```python
from build123d import *

# Parameters (mm, degrees)
SKETCH1_R           = 9
BOSS_EXTRUDE1_DEPTH = 70
SKETCH2_R           = 2.5
CUT_EXTRUDE1_DEPTH  = 15
CUT_EXTRUDE2_START  = -50
SKETCH3_R           = 9
SKETCH3_R_2         = 7.5
CUT_EXTRUDE2_DEPTH  = 50
FILLET1_R           = 10


with BuildPart() as part:
    # Sketch1 → Boss-Extrude1 (new body)
    with BuildSketch(Plane.XY):
        Circle(SKETCH1_R)
    extrude(amount=BOSS_EXTRUDE1_DEPTH)

    # Sketch2 → Cut-Extrude1 (cut)
    with BuildSketch(Plane(origin=(0, 0, 0), x_dir=(-1, 0, 0), z_dir=(0, 0, -1))):
        Circle(SKETCH2_R)
    extrude(amount=-CUT_EXTRUDE1_DEPTH, mode=Mode.SUBTRACT)

    # Sketch3 → Cut-Extrude2 (cut)
    with BuildSketch(Plane.XY.offset(70).offset(CUT_EXTRUDE2_START)):
        Circle(SKETCH3_R)
        Circle(SKETCH3_R_2, mode=Mode.SUBTRACT)
    extrude(amount=CUT_EXTRUDE2_DEPTH, mode=Mode.SUBTRACT)

    # Fillet1
    # the kernel refuses this fillet: 10 mm, written as the material it adds along each edge
    with BuildSketch(Plane(origin=(0, 0, 20), x_dir=(1, 0, 0), z_dir=(0, -1, 0))) as fillet1_piece_1:
        with BuildLine():
            CenterArc((17.5, 5.267826876), FILLET1_R, 180, 31.788330617)
            Line((7.5, 5.267826876), (7.3, 5.267826876))
            Line((7.3, 5.267826876), (7.3, 0))
            Line((7.3, 0), (7.5, -0.2))
            ThreePointArc((7.5, -0.2), (8.25, -0.2), (8.83, -0.105356538))
            Line((8.83, -0.105356538), (9, 0))
        make_face()
    revolve(axis=Axis((0, 0, 20), (0, 0, 1)))


solid = part.part
```
Model file for the job. Use its own axes, mm. A direction names the side the tool comes from. Coordinates: 2 decimals unless noted, no trailing zeros. Write each loop counter-clockwise with the first axis right and the second up, starting at its lowest first coordinate (ties: lowest second). Pieces come first, ordered by that corner, then holes. Notation, with made-up numbers: (15, 42.5) - (20, 42.5) arc R23 cw to (20, 79.5) - close; hole circle Ø10 at (4, 41.25). An arc over 180 degrees is marked (long way). One line per question, with ' | ' between items. Start each with the question number.
Q1. Cut at A-A, the plane y = 0. List the corners of the cut face in (x, z).
Q2. Drill centre lines: line 1 (Y direction, x = 0, z = 8.5); line 2 (Z direction, x = 1.25, y = -2); line 3 (X direction, y = -2, z = 7.5). Where is each one in solid material? Low to high. Write a range as [from, to].
Q3. Pull direction X, two halves, no side cores. Call faces 3 (the face through (-7.493, 0.33, 47.321)), 4 (the face through (2, -2, 0)), 5 (the face through (0, 0, 15)): pulls with the +X half, pulls with the -X half, needs draft (parallel to the pull), parting line crosses it, or undercut.
Q4. Cut at C-C, the plane z = 66.5. List the corners of the cut face in (x, y).
Q5. Cut at D-D, the plane z = 10.5. List the corners of the cut face in (x, y), then the cut area to 3 significant figures.
Q6. Pin check, flat tips, straight feed: pin 1 (2 mm diameter, centred on y = 6.5, z = 46.5, fed in from +X); pin 2 (1 mm diameter, centred on x = -3, z = 61, fed in from +Y); pin 3 (5 mm diameter, centred on y = 0.5, z = 37.5, fed in from -X); pin 4 (6 mm diameter, centred on x = 0, y = 0, fed in from -Z). Stop position of each tip, or through.
Q7. 3-axis set-ups, long thin cutter, end or side, ignore diameter. For faces 1 (the face through (0.54, -2.44, 7.4)), 2 (the face through (0, 0, 70)): which of +Z, -Z, +X, -X, +Y, -Y reach the whole face in a straight line?
Answer below:
1) outline: (-9, 0) - (-2.5, 0) - (-2.5, 15) - (2.5, 15) - (2.5, 0) - (9, 0) - (9, 20) arc R10 cw to (7.5, 25.27) - (7.5, 70) - (-7.5, 70) - (-7.5, 25.27) arc R10 cw to (-9, 20) - close
2) line 1: [-9, -2.5], [2.5, 9] | line 2: [15, 70] | line 3: [-8.77, -1.5], [1.5, 8.77]
3) face 3: parting line crosses it | face 4: needs draft | face 5: undercut
4) outline: circle Ø15 at (0, 0)
5) outline: circle Ø18 at (0, 0); hole circle Ø5 at (0, 0) | area: 235 mm^2
6) pin 1: x = 5.1 | pin 2: y = 7.07 | pin 3: x = -7.5 | pin 4: z = 0
7) face 1: -Z | face 2: +Z, +X, -X, +Y, -Y
